Geometry check sheet. Reference: the model listing, model coordinates, mm. A direction names the side the tool comes from. Round coordinates to 2 decimals unless told otherwise and drop trailing zeros. Order: outer loops, then holes, each group sorted by start corner. A loop starts at its lowest first (then second) coordinate and runs counter-clockwise, first axis right, second up.
(1) Gauge pin test, flat ends, axial feed: P1, Ø8, axis at x = -23.5, z = 15, coming from the +Y side; P2, Ø7.5, axis at y = 13.16, z = 7.42, coming from the -X side; P3, Ø5.5, axis at x = -16.129, z = 31.115, coming from the -Y side; P4, Ø2, axis at y = 8.5, z = 21.5, coming from the -X side. Record the tip position at first contact, or that the pin passes through.
(2) Thickness scan on L1, parallel to Y at x = -32, z = 20.5; L2, parallel to X at y = 16.5, z = 10; L3, parallel to Y at x = -4, z = 19. Record the ranges inside material, lowest first.
(3) Cross-section at B-B on z = 16.5. Enter the section's corners in (x, y), and give its area (3 significant figures).
(4) Cross-section at D-D on z = 12.5. Enter the section's corners in (x, y), and give its area (3 significant figures).
(5) Set-up check for faces 4 (the face through (-27.491, 2.88, 33.214)), 5 (the face through (-5.842, 28, 18)): record each of +Z, -Z, +X, -X, +Y, -Y from which the full face is reachable in a straight line by a thin tool's end or side.
(6) Cross-section at C-C on x = -16.5. Enter the section's corners in (y, z).
(7) Cross-section at A-A on y = 19.5. Enter the section's corners in (x, z), and give its area (3 significant figures).
(8) Draft check along Y on faces 1 (the face through (-25, 5.842, 18)), 2 (the face through (-2.88, 29.69, 16.48)), 3 (the face through (-26.455, 2.88, 6.463)). Enter one of: pulls with the +Y half, pulls with the -Y half, needs draft (parallel to the pull), parting line crosses it, or undercut.
from build123d import *

# Parameters (mm, degrees)
BOSS_EXTRUDE1_DEPTH = 36.83
SKETCH2_R           = 7.14375
SKETCH2_R_2         = 3.175
CUT_EXTRUDE1_DEPTH  = 66.682081939
SKETCH3_R           = 2.4892
CUT_EXTRUDE2_DEPTH  = 66.682081995


with BuildPart() as part:
    # Sketch1 → Boss-Extrude1 (new body)
    with BuildSketch(Plane.XY):
        with BuildLine():
            Line((0, 38.5572), (0, 0))
            Line((0, 0), (-38.354, 0))
            Line((-38.354, 0), (-38.354, 5.842))
            Line((-38.354, 5.842), (-10.922, 5.842))
            ThreePointArc((-10.922, 5.842), (-7.329897552, 7.329897552), (-5.842, 10.922))
            Line((-5.842, 10.922), (-5.842, 38.5572))
            Line((-5.842, 38.5572), (0, 38.5572))
        make_face()
    extrude(amount=BOSS_EXTRUDE1_DEPTH)

    # Sketch2 → Cut-Extrude1 (cut, through all)
    with BuildSketch(Plane(origin=(0, 0, 0), x_dir=(0, 0, -1), z_dir=(1, 0, 0))):
        with Locations(Location((-18.415, 19.5072, 0), (0, 0, 90))):
            Circle(SKETCH2_R)
        with Locations(Location((-18.415, 32.2072, 0), (0, 0, 90))):
            Circle(SKETCH2_R_2)
        with Locations(Location((-7.416477372, 13.1572, 0), (0, 0, 90))):
            Circle(SKETCH2_R_2)
        with Locations(Location((-29.413522628, 13.1572, 0), (0, 0, 90))):
            Circle(SKETCH2_R_2)
    extrude(amount=-CUT_EXTRUDE1_DEPTH, mode=Mode.SUBTRACT)

    # Sketch3 → Cut-Extrude2 (cut, through all)
    with BuildSketch(Plane.XZ):
        with Locations((-28.829, 31.115)):
            Circle(SKETCH3_R)
        with Locations((-16.129, 31.115)):
            Circle(SKETCH3_R)
        with Locations((-16.129, 5.715)):
            Circle(SKETCH3_R)
        with Locations((-28.829, 5.715)):
            Circle(SKETCH3_R)
    extrude(amount=-CUT_EXTRUDE2_DEPTH, mode=Mode.SUBTRACT)


solid = part.part
Found:
1. P1: stops at y = 5.84
1. P2: stops at x = -6.07
1. P3: stops at y = 0
1. P4: stops at x = -7.17
2. L1: y = 0 to 5.84
2. L2: x = -5.84 to 0
2. L3: y = 0 to 12.39, 26.63 to 29.09, 35.33 to 38.56
3. outline: (-38.35, 0) - (0, 0) - (0, 12.62) - (-5.84, 12.62) - (-5.84, 10.92) arc R5.08 cw to (-10.92, 5.84) - (-38.35, 5.84) - close; (-5.84, 26.39) - (0, 26.39) - (0, 29.67) - (-5.84, 29.67) - close; (-5.84, 34.74) - (0, 34.74) - (0, 38.56) - (-5.84, 38.56) - close
3. area: 311 mm2
4. outline: (-38.35, 0) - (0, 0) - (0, 15.5) - (-5.84, 15.5) - (-5.84, 10.92) arc R5.08 cw to (-10.92, 5.84) - (-38.35, 5.84) - close; (-5.84, 23.51) - (0, 23.51) - (0, 38.56) - (-5.84, 38.56) - close
4. area: 374 mm2
5. face 4: +Y, -Y
5. face 5: +Z, -Z, -X, +Y
6. outline: (0, 0) - (5.84, 0) - (5.84, 3.25) - (0, 3.25) - close; (0, 8.18) - (5.84, 8.18) - (5.84, 28.65) - (0, 28.65) - close; (0, 33.58) - (5.84, 33.58) - (5.84, 36.83) - (0, 36.83) - close
7. outline: (-5.84, 0) - (0, 0) - (0, 11.27) - (-5.84, 11.27) - close; (-5.84, 25.56) - (0, 25.56) - (0, 36.83) - (-5.84, 36.83) - close
7. area: 132 mm2
8. face 1: pulls with the +Y half
8. face 2: undercut
8. face 3: needs draft
